Can you work these out from the model? Positions are in its coordinate system, mm. Give positions to 0.01 mm unless a question says otherwise; leave off trailing zeros. Loops run counter-clockwise (first coordinate to the right, second up) from the corner with the lowest first, then second, coordinate; pieces in that order, holes last.
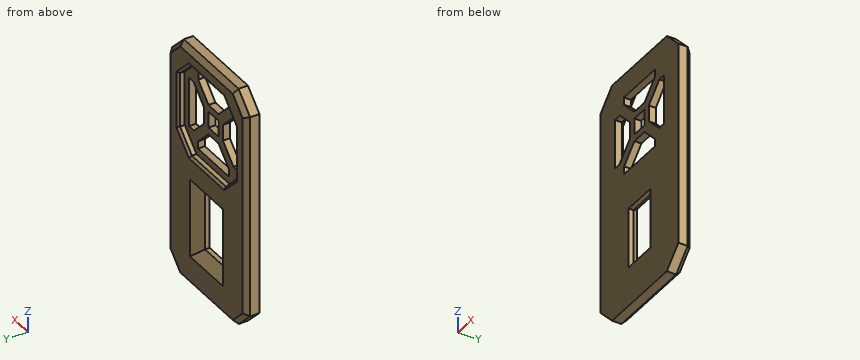
Autodesk Inventor part; units mm, degrees
ref_plane "YZ Plane" through (0, 0, 0) normal (1, 0, 0) x (0, 1, 0)
ref_plane "XZ Plane" through (0, 0, 0) normal (0, 1, 0) x (-1, 0, 0)
ref_plane "XY Plane" through (0, 0, 0) normal (0, 0, 1) x (1, 0, 0)
sketch "Sketch1" plane through (0, 0, 0) normal (0, 1, 0) x (-1, 0, 0)
  line L0 (-20, 20) -> (20, 20)
  line L1 (20, 20) -> (20, -20)
  line L2 (20, -20) -> (-20, -20)
  line L3 (-20, -20) -> (-20, 20)
  line L4 (-20, 20) -> (20, -20) construction
  line L5 (20, 20) -> (-20, -20) construction
  line L6 (27, 27) -> (-27, 27)
  line L7 (-27, 27) -> (-27, -77)
  line L8 (-27, -77) -> (27, -77)
  line L9 (27, -77) -> (27, 27)
  line L10 (27, -27) -> (-27, -27)
  line L11 (7.5, -39) -> (-7.5, -39)
  line L12 (-7.5, -39) -> (-7.5, -65)
  line L13 (-7.5, -65) -> (7.5, -65)
  line L14 (7.5, -65) -> (7.5, -39)
  line L15 (-27, 19) -> (-19, 27)
  line L16 (27, 19) -> (19, 27)
  line L17 (0, -31.8198) -> (-31.8198, 0)
  line L18 (-31.8198, 0) -> (0, 31.8198)
  line L19 (0, 31.8198) -> (31.8198, 0)
  line L20 (31.8198, 0) -> (0, -31.8198)
  line L21 (0, -31.8198) -> (0, 31.8198) construction
  line L22 (-31.8198, 0) -> (31.8198, 0) construction
  line L23 (-19, -77) -> (-27, -69)
  line L24 (27, -69) -> (19, -77)
  point P0 (0, 0)
  point P1 (20, 0)
  point P2 (0, -27)
  point P3 (0, -65)
  point P4 (-7.5, -52)
  point P5 (-20, -11.8198)
  point P6 (-20, 11.8198)
  point P7 (-11.8198, 20)
  point P8 (11.8198, 20)
  point P9 (20, 11.8198)
  point P10 (20, -11.8198)
  point P11 (11.8198, -20)
  point P12 (-11.8198, -20)
  dimension "d0" = 40
  dimension "d1" = 40
  dimension "d2" = 7
  dimension "d3" = 7
  dimension "d4" = 7
  dimension "d5" = 7
  dimension "d6" = 50
  dimension "d7" = 0
  dimension "d8" = 25
  dimension "d9" = 26
  dimension "d10" = 15
  dimension "d11" = 45
  dimension "d12" = 135
  dimension "d13" = 45
  dimension "d14" = 8
  dimension "d15" = 135
  dimension "d16" = 8
  dimension "d21" = 135
  dimension "d22" = 8
  dimension "d23" = 8
extrude "Extrusion1" add sketch "Sketch1" along normal blind 4 and the other way blind 2 contours L3 L18 L7 L15 L6 L0 | L0 L18 L3 | L18 L6 L19 L0 | L0 L19 L1 L20 L2 L17 L3 L18 | L3 L17 L7 L18 | L19 L6 L16 L9 L1 L0 | L0 L1 L19 | L17 L2 L3 | L3 L2 L17 L10 L7 | L19 L9 L20 L1 | L2 L20 L10 L17 | L20 L9 L10 L2 L1 | L1 L2 L20 | L17 L20 L10 L9 L24 L8 L23 L7 | L10 L20 L17 | L14 L13 L12 L11
sketch "Sketch8" plane through (0, 4, 0) normal (0, 1, 0) x (1, 0, 0)
  line L0 (7.5, 70) -> (7.5, 44)
  line L1 (-7.5, 44) -> (-7.5, 70)
  line L2 (7.5, 70) -> (-7.5, 70)
  line L3 (-7.5, 70) -> (-7.5, 44)
  line L4 (-7.5, 44) -> (7.5, 44)
  line L5 (7.5, 44) -> (7.5, 70)
  line L6 (-20, 20) -> (20, 20)
  line L7 (20, 20) -> (20, -20)
  line L8 (20, -20) -> (-20, -20)
  line L9 (-20, -20) -> (-20, 20)
  line L10 (20, 11.8198) -> (20, -11.8198)
  line L11 (11.8198, -20) -> (-11.8198, -20)
  line L12 (-20, -11.8198) -> (-20, 11.8198)
  line L13 (-11.8198, 20) -> (11.8198, 20)
  line L14 (20, 11.8198) -> (11.8198, 20)
  line L15 (20, 11.8198) -> (11.8198, 20)
  line L16 (20, -11.8198) -> (20, 11.8198)
  line L17 (20, -11.8198) -> (11.8198, -20)
  line L18 (20, -11.8198) -> (11.8198, -20)
  line L19 (-20, -11.8198) -> (-11.8198, -20)
  line L20 (-11.8198, 20) -> (-20, 11.8198)
  point P0 (0, 0)
  point P1 (-11.8198, -20)
  point P2 (11.8198, 20)
  dimension "d35" = 0
  dimension "d36" = 0
  dimension "d37" = 0
  dimension "d38" = 0
extrude "Extrusion3" cut sketch "Sketch8" against normal blind 3 contours L6 L14 L7 L17 L8 L19 L9 L20
sketch "Sketch10" plane through (0, 4, 0) normal (0, 1, 0) x (1, 0, 0)
  line L0 (7.5, 60) -> (-7.5, 60)
  line L1 (-7.5, 60) -> (-7.5, 34)
  line L2 (-7.5, 34) -> (7.5, 34)
  line L3 (7.5, 34) -> (7.5, 60)
  line L4 (19, 77) -> (-19, 77)
  point P0 (0, 0)
  point P1 (0, 77)
  point P2 (0, 34)
  point P3 (7.5, 47)
  dimension "d41" = 0
  dimension "d42" = 15
  dimension "d43" = 26
  dimension "d44" = 30
extrude "Extrusion4" cut sketch "Sketch10" against normal through all
chamfer "Chamfer1" distance 4 angle 45 4 edges at (7.5, 4, -47) (0, 4, -60) (-7.5, 4, -47) (0, 4, -34)
sketch "Sketch11" plane through (0, 1, 0) normal (0, 1, 0) x (1, 0, 0)
  line L0 (-3.5, 3.5) -> (3.5, 3.5)
  line L1 (3.5, 3.5) -> (3.5, -3.5)
  line L2 (3.5, -3.5) -> (-3.5, -3.5)
  line L3 (-3.5, -3.5) -> (-3.5, 3.5)
  line L4 (-3.5, 3.5) -> (3.5, -3.5) construction
  line L5 (3.5, 3.5) -> (-3.5, -3.5) construction
  line L6 (17, 10.6132) -> (17, -10.818)
  line L7 (20, 11.8198) -> (20, -11.8198)
  line L8 (6.5, 3.5) -> (6.5, -3.5)
  line L9 (17, 10.6132) -> (10.2264, 10.6132)
  line L10 (17, -10.818) -> (11.4927, -10.818)
  line L11 (6.5, -3.5) -> (13.818, -10.818)
  line L12 (6.5, 3.5) -> (13.6132, 10.6132)
  line L13 (20, -11.8198) -> (11.8198, -20)
  line L14 (11.8198, 20) -> (20, 11.8198)
  point P0 (0, 0)
  point P1 (6.5, 0)
  point P2 (3.5, 0)
  dimension "d50" = 7
  dimension "d51" = 7
  dimension "d52" = 3
  dimension "d53" = 3
  dimension "d54" = 0
  dimension "d55" = 7
extrude "Extrusion5" cut sketch "Sketch11" against normal through all
pattern_circular "Circular Pattern1" count 4 over 360 about axis through (0, -10, 0) along (0, 1, 0) of "Extrusion5"
chamfer "Chamfer2" distance 2 angle 45 8 edges at (-27, 4, -25) (-23, 4, -73) (0, 4, -77) (23, 4, -73) (27, 4, -25) (23, 4, 23) (0, 4, 27) (-23, 4, 23)
chamfer "Chamfer3" distance 1 angle 45 8 edges at (20, 4, 0) (15.9099, 4, -15.9099) (0, 4, -20) (-15.9099, 4, -15.9099) (-20, 4, 0) (-15.9099, 4, 15.9099) (0, 4, 20) (15.9099, 4, 15.9099)
properties part number "front_pannel_v2"
(1) Suppose I cut it at C-C on z = 4.5. List the corners of the cut face in (x, y) for me.
Returned:
outline: (-27, -2) - (-17, -2) - (-17, 1) - (-20, 1) - (-20, 3) - (-21, 4) - (-25, 4) - (-27, 2) - close; (-7.5, -2) - (7.5, -2) - (7.5, 1) - (-7.5, 1) - close; (17, -2) - (27, -2) - (27, 2) - (25, 4) - (21, 4) - (20, 3) - (20, 1) - (17, 1) - close
(2) Suppose I cut it at D-D on z = -33. List the corners of the cut face in (x, y) for me, plus the area to 3 significant figures.
Returned:
outline: (-27, -2) - (27, -2) - (27, 2) - (25, 4) - (11.5, 4) - (8.5, 1) - (-8.5, 1) - (-11.5, 4) - (-25, 4) - (-27, 2) - close
area: 260 mm2
(3) Please list where these lines run through material, in increasing order: probe 1 along X at (y, z) = (0.5, 0); probe 2 along Z at (x, y) = (-0.5, 3); probe 3 along X at (y, z) = (0, -7).
Returned:
probe 1: x = -27 to -17, -6.5 to -3.5, 3.5 to 6.5, 17 to 27
probe 2: z = -76 to -63, -31 to -20, 20 to 26
probe 3: x = -27 to -17, -10 to -4, 4 to 10, 17 to 27
(4) Suppose I cut it at B-B on x = 9. List the corners of the cut face in (y, z) for me.
Returned:
outline: (-2, -77) - (2, -77) - (4, -75) - (4, -64) - (1.5, -61.5) - (1.5, -32.5) - (4, -30) - (4, -21) - (3, -20) - (1, -20) - (1, -17) - (-2, -17) - close; (-2, -12) - (1, -12) - (1, -6) - (-2, -6) - close; (-2, 6) - (1, 6) - (1, 12) - (-2, 12) - close; (-2, 17) - (1, 17) - (1, 20) - (3, 20) - (4, 21) - (4, 25) - (2, 27) - (-2, 27) - close
(5) Suppose I cut it at A-A on z = -47. List the corners of the cut face in (x, y) for me.
Returned:
outline: (-27, -2) - (-7.5, -2) - (-7.5, 0) - (-11.5, 4) - (-25, 4) - (-27, 2) - close; (7.5, -2) - (27, -2) - (27, 2) - (25, 4) - (11.5, 4) - (7.5, 0) - close
(6) Will these pins go through, and if not, where does the flat tip stop? P1, Ø6, axis at x = -4, z = -45, coming from the +Y side; P2, Ø6, axis at x = 5, z = -55, coming from the -Y side.
Returned:
P1: passes through
P2: stops at y = -2
